```python
from build123d import *

# Parameters (mm, degrees)
SKETCH1_W           = 500
SKETCH1_H           = 98.65
BOSS_EXTRUDE1_DEPTH = 12
SKETCH2_W           = 12
SKETCH2_H           = 24
SKETCH2_W_2         = 333.333333334
SKETCH2_H_2         = 12
CUT_EXTRUDE1_DEPTH  = 510.78017076
SCALE1_SCALE        = 0.5
SKETCH3_W           = 38.5
SKETCH3_H           = 15
CUT_EXTRUDE2_DEPTH  = 383.276274645
FILLET1_R           = 7


with BuildPart() as part:
    # Sketch1 → Boss-Extrude1 (new body)
    with BuildSketch(Plane.XY):
        with Locations((250, 49.325)):
            Rectangle(SKETCH1_W, SKETCH1_H)
    extrude(amount=BOSS_EXTRUDE1_DEPTH)

    # Sketch2 → Cut-Extrude1 (cut, through all)
    with BuildSketch(Plane.XY.offset(12)):
        with Locations((494, 86.65)):
            Rectangle(SKETCH2_W, SKETCH2_H)
        with Locations((494, 12)):
            Rectangle(SKETCH2_W, SKETCH2_H)
        with Locations((6, 12)):
            Rectangle(SKETCH2_W, SKETCH2_H)
        with Locations((6, 86.65)):
            Rectangle(SKETCH2_W, SKETCH2_H)
        with Locations((250, 92.65)):
            Rectangle(SKETCH2_W_2, SKETCH2_H_2)
        with Locations((250, 6)):
            Rectangle(SKETCH2_W_2, SKETCH2_H_2)
    extrude(amount=-CUT_EXTRUDE1_DEPTH, mode=Mode.SUBTRACT)


with BuildPart() as part_1:
    # Scale1: scaled about (250, 49.325, 6)
    add(part.part.scale(SCALE1_SCALE).moved(Location((125, 24.6625, 3))))

    # Sketch3 → Cut-Extrude2 (cut, through all)
    with BuildSketch(Plane.XY.offset(9)):
        with Locations((310.253333333, 38.1625)):
            Rectangle(SKETCH3_W, SKETCH3_H)
        with Locations((255.753333333, 38.1625)):
            Rectangle(SKETCH3_W, SKETCH3_H)
    extrude(amount=-CUT_EXTRUDE2_DEPTH, mode=Mode.SUBTRACT)

    # Fillet1
    fillet1_edges = [part_1.edges().sort_by_distance(p)[0] for p in [
        (329.503333333, 45.6625, 6),
        (275.003333333, 45.6625, 6),
    ]]
    fillet(fillet1_edges, radius=FILLET1_R)


solid = part_1.part
```
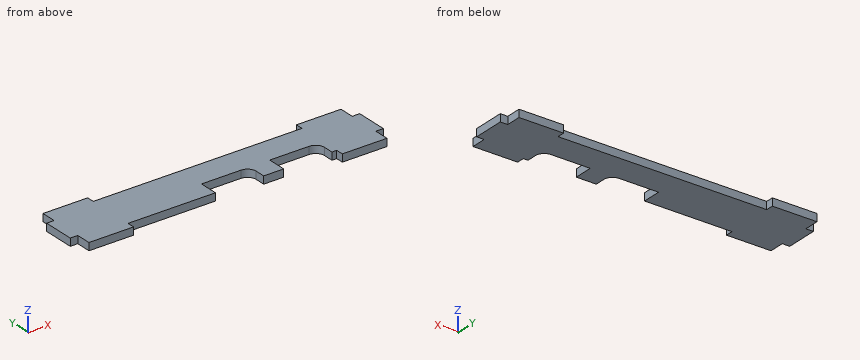
Check sheet for the modelled part. Datum: model origin and axes. Units: mm. Round coordinates to 2 decimals unless told otherwise and drop trailing zeros. Loops run counter-clockwise (first coordinate to the right, second up) from the corner with the lowest first, then second, coordinate; pieces in that order, holes last. Notation, with made-up numbers: (67.25, 47.5) - (102.25, 47.5) arc R17 cw to (102.25, 52.5) - close; hole circle Ø10 at (-12.5, 67). An arc over 180 degrees is marked (long way). Write item = value, one per line. Start each with the question number.
Q1. Section check A-A (y = 33.5). Record the boundary of the cut face in (x, z), plus the area to 3 significant figures.
Q2. Depth check by flat-ended pin: P1, Ø1.8, axis at y = 35.5, z = 6, coming from the -X side; P2, Ø1.9, axis at x = 331.5, z = 5.5, coming from the -Y side; P3, Ø1.8, axis at x = 373.5, z = 7, coming from the +Y side. Enter the tip coordinate at first touch or a pass-through.
Q3. Section check C-C (x = 315). Record the boundary of the cut face in (y, z).
Q4. Thickness scan on L1, parallel to X at y = 33.5, z = 6.5; L2, parallel to X at y = 37.5, z = 6.6; L3, parallel to X at y = 70.5, z = 6.75. Record the ranges inside material, lowest first.
Q5. Section check D-D (y = 42.5). Record the boundary of the cut face in (x, z), plus the area to 3 significant figures.
Derived:
q1.outline = (131, 3) - (236.5, 3) - (236.5, 9) - (131, 9) - close; (275, 3) - (291, 3) - (291, 9) - (275, 9) - close; (329.5, 3) - (369, 3) - (369, 9) - (329.5, 9) - close
q1.area = 966 mm^2
q2.P1 = 131
q2.P2 = 30.66
q2.P3 = 61.99
q3.outline = (45.66, 3) - (67.99, 3) - (67.99, 9) - (45.66, 9) - close
q4.L1 = 131 to 236.5, 275 to 291, 329.5 to 369
q4.L2 = 125 to 236.5, 275 to 291, 329.5 to 375
q4.L3 = 131 to 166.67, 333.33 to 369
q5.outline = (125, 3) - (236.5, 3) - (236.5, 9) - (125, 9) - close; (273.86, 3) - (291, 3) - (291, 9) - (273.86, 9) - close; (328.36, 3) - (375, 3) - (375, 9) - (328.36, 9) - close
q5.area = 1,050 mm^2
